Autodesk Inventor part; units mm, degrees
ref_plane "YZ Plane" through (0, 0, 0) normal (1, 0, 0) x (0, 1, 0)
ref_plane "XZ Plane" through (0, 0, 0) normal (0, 1, 0) x (-1, 0, 0)
ref_plane "XY Plane" through (0, 0, 0) normal (0, 0, 1) x (1, 0, 0)
sketch "Skizze1" plane through (0, 0, 0) normal (0, 0, 1) x (1, 0, 0)
  line L0 (-71.5, 15.5) -> (71.5, 15.5)
  line L1 (71.5, 15.5) -> (71.5, -15.5)
  line L2 (71.5, -15.5) -> (-71.5, -15.5)
  line L3 (-71.5, -15.5) -> (-71.5, 15.5)
  line L4 (0, -21.7) -> (0, 21.7)
  line L5 (-100.1, 0) -> (100.1, 0)
  point P0 (0, 0)
  dimension "d0" = 143
  dimension "d1" = 31
extrude "Extrusion1" add sketch "Skizze1" against normal mid plane 43
sketch "Skizze2" plane through (-71.5, 15.5, -21.5) normal (0, 1, 0) x (1, 0, 0)
  line L0 (4, -4) -> (139, -4)
  line L1 (139, -4) -> (139, -39)
  line L2 (139, -39) -> (4, -39)
  line L3 (4, -39) -> (4, -4)
  line L4 (143, -43) -> (0, -43)
  line L5 (0, 0) -> (143, 0)
  line L6 (0, 0) -> (0, -43)
  line L7 (143, 0) -> (143, -43)
  point P0 (71.5, -21.5)
  dimension "d5" = 4
  dimension "d6" = 4
  dimension "d7" = 4
  dimension "d8" = 4
extrude "Extrusion2" add sketch "Skizze2" along normal blind 0.2 contours L0 L1 L2 L3
sketch "Skizze3" plane through (71.5, -15.5, -21.5) normal (1, 0, 0) x (0, 0, -1)
  circle A0 centre (-5, 26) radius 2.5
  line L0 (0, 31) -> (-43, 31)
  line L1 (0, 31) -> (0, 0)
  circle A1 centre (-5, 20.5) radius 2.5
  point P0 (-21.5, 15.5)
  dimension "d11" = 5
  dimension "d12" = 5
  dimension "d13" = 5
  dimension "d14" = 5
  dimension "d15" = 5
  dimension "d16" = 5.5
extrude "Extrusion3" add sketch "Skizze3" along normal blind 20
properties part number "Akku"
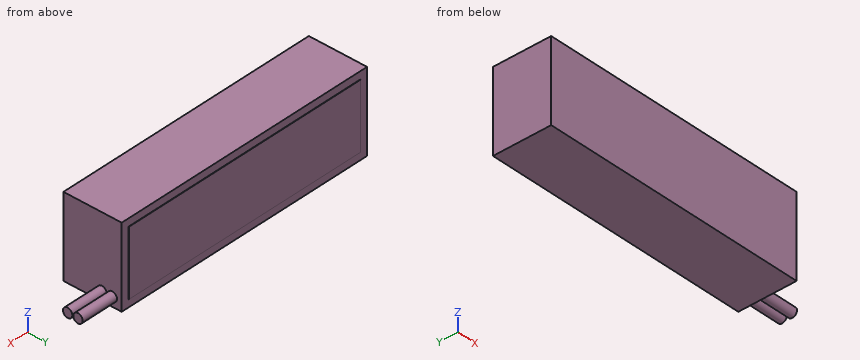
Verification items for the finished model (mm, model axes). Give positions to 0.01 mm unless a question says otherwise; leave off trailing zeros. Order: outer loops, then holes, each group sorted by start corner. A loop starts at its lowest first (then second) coordinate and runs counter-clockwise, first axis right, second up. Notation, with made-up numbers: M 76.5,-7.75 L 112.5,-7.75 A18 cw 112.5,22.25 Z; hole C 60,82.5 d4. An arc over 180 degrees is marked long. Return JSON: item names as keys, results as strings. Group by question number.
1) Section check A-A on z = -2. Record the cut outline in (x, y), and give its area (3 significant figures).
2) Section check C-C on y = -7.5. Record the cut outline in (x, z), and give its area (3 significant figures).
3) Section check B-B on y = 10.5. Record the cut outline in (x, z), and give its area (3 significant figures).
4) Go/stop test with a flat-tipped pin: pin 1 Ø6 at (y, z) = (5, 5.5) entering from +X. Record where the tip stops, or that it passes through.
5) Section check D-D on z = 19.5. Record the cut outline in (x, y).
6) Scan lines: line 1 (X direction, y = 13.5, z = -13); line 2 (Y direction, x = -52.5, z = 18.5); line 3 (Z direction, x = 75, y = 7). Record each from-to range of solid material in increasing order.
Answer block:
{
 "1": {"outline": "M -71.5,-15.5 L 71.5,-15.5 L 71.5,15.5 L 67.5,15.5 L 67.5,15.7 L -67.5,15.7 L -67.5,15.5 L -71.5,15.5 Z", "area": "4,460 mm^2"},
 "2": {"outline": "M -71.5,-21.5 L 71.5,-21.5 L 71.5,21.5 L -71.5,21.5 Z", "area": "6,150 mm^2"},
 "3": {"outline": "M -71.5,-21.5 L 71.5,-21.5 L 71.5,-19 L 91.5,-19 L 91.5,-14 L 71.5,-14 L 71.5,21.5 L -71.5,21.5 Z", "area": "6,250 mm^2"},
 "4": {"pin 1": "stops at x = 71.5"},
 "5": {"outline": "M -71.5,-15.5 L 71.5,-15.5 L 71.5,15.5 L -71.5,15.5 Z"},
 "6": {"line 1": "x = -71.5 to 71.5", "line 2": "y = -15.5 to 15.5", "line 3": "z = -18 to -15"}
}
